The model under review builds one solid part; all positions refer to its coordinate system, in mm. A direction names the side the tool comes from. Give positions to 0.01 mm unless a question says otherwise; leave off trailing zeros. Order: outer loops, then holes, each group sorted by start corner. A loop starts at its lowest first (then second) coordinate and runs counter-clockwise, first axis right, second up.
Solid Edge part; units mm, degrees
sketch "Sketch1" plane through (0, 0, 0) normal (0, 0, 1) x (1, 0, 0)
  line L0 (70, 0) -> (70, 165)
  line L1 (70, 165) -> (0, 165)
  line L2 (0, 165) -> (0, 0)
  line L3 (0, 0) -> (70, 0)
extrude "Protrusion1" add sketch "Sketch1" along normal blind 4
sketch "Sketch2" plane through (35, 82.5, 4) normal (0, 0, 1) x (0, 1, 0)
  line L0 (78.5, 31) -> (-78.5, 31)
  line L1 (-78.5, 31) -> (-78.5, -31)
  line L2 (-78.5, -31) -> (78.5, -31)
  line L3 (78.5, -31) -> (78.5, 31)
  line L4 (-82.5, -35) -> (82.5, -35)
  line L5 (82.5, -35) -> (82.5, 35)
  line L6 (82.5, 35) -> (-82.5, 35)
  line L7 (-82.5, 35) -> (-82.5, -35)
extrude "ProtrusiónExtruida_2" add sketch "Sketch2" along normal blind 100
Item 1: Take a section at B-B (x = 19). Give the boundary of the cut face in (y, z), and give its area (3 significant figures).
Values found:
outline: (0, 0) - (165, 0) - (165, 104) - (161, 104) - (161, 4) - (4, 4) - (4, 104) - (0, 104) - close
area: 1,460 mm2
Item 2: Take a section at A-A (z = 51). Give the boundary of the cut face in (x, y).
Values found:
outline: (0, 0) - (70, 0) - (70, 165) - (0, 165) - close; hole (4, 4) - (66, 4) - (66, 161) - (4, 161) - close
Item 3: Take a section at C-C (y = 91.5). Give the boundary of the cut face in (x, z).
Values found:
outline: (0, 0) - (70, 0) - (70, 104) - (66, 104) - (66, 4) - (4, 4) - (4, 104) - (0, 104) - close
Item 4: Draft analysis for pull direction X (two halves, no side actions). For faces 1 (the flat face through (70, 81, 51)), 2 (the flat face through (4, 84, 53)), 3 (the flat face through (35, 165, 51)), 4 (the flat face through (0, 84, 51)), state which applies: released by +X, released by -X, zero draft, split by the parting line, or undercut.
Values found:
face 1: released by +X
face 2: undercut
face 3: zero draft
face 4: released by -X
Item 5: For faces 5 (the flat face through (35, 0, 51)), 6 (the flat face through (35, 4, 53)), list the 3-axis set-ups (+Z, -Z, +X, -X, +Y, -Y) from which the entire face can be reached by the end or side of a thin tool; tool diameter is ignored.
Values found:
face 5: +Z, -Z, +X, -X, -Y
face 6: +Z
Item 6: Clearance check with a flat-ended pin moving along its axis: pin 1 Ø3 at (x, y) = (18, 27) entering from +Z. State where the tip first meets the part, or that it passes through.
Values found:
pin 1: stops at z = 4
Item 7: For line 1 (Y direction, x = 9.5, z = 48); line 2 (X direction, y = 113.5, z = 20); line 3 (Z direction, x = 59, y = 151.5), list the stretches that pass through material, from the lowest coordinate up.
Values found:
line 1: y = 0 to 4, 161 to 165
line 2: x = 0 to 4, 66 to 70
line 3: z = 0 to 4
